from build123d import *

# Parameters (mm, degrees)
SKETCH1_R               = 6.35
BOSS_EXTRUDE1_DEPTH     = 25.4
SHELL1_T                = -0.889
FILLET1_R               = 1.27
SKETCH2_R               = 4.7625
BOSS_EXTRUDE2_DEPTH     = 10.16
CUT_EXTRUDE1_START      = -10.16
CUT_EXTRUDE1_DEPTH      = 10.16
CUT_EXTRUDE2_DEPTH      = 28.452277251
CUT_EXTRUDE2_DEPTH_BACK = 28.452277251
SKETCH4_R               = 3.048
CHAMFER2_SIZE           = 0.381
FILLET2_R               = 1.27


with BuildPart() as part:
    # Sketch1 → Boss-Extrude1 (new body)
    with BuildSketch(Plane.XY):
        Circle(SKETCH1_R)
    extrude(amount=BOSS_EXTRUDE1_DEPTH)

    # Shell1
    shell1_openings = [part.faces().sort_by_distance(p)[0] for p in [
        (0, 0, 25.4),
    ]]
    offset(amount=SHELL1_T, openings=shell1_openings, kind=Kind.INTERSECTION)

    # Fillet1
    fillet1_edges = [part.edges().sort_by_distance(p)[0] for p in [
        (-6.35, 0, 0),
    ]]
    fillet(fillet1_edges, radius=FILLET1_R)

    # Sketch2 → Boss-Extrude2 (add)
    with BuildSketch(Plane(origin=(0, 0, 0), x_dir=(-1, 0, 0), z_dir=(0, 0, -1))):
        with Locations(Location((0, 0, 0), (0, 0, 180))):
            Circle(SKETCH2_R)
    extrude(amount=BOSS_EXTRUDE2_DEPTH)

    # Sketch3 → Cut-Extrude1 (cut)
    with BuildSketch(Plane(origin=(0, 0, -10.16), x_dir=(-1, 0, 0), z_dir=(0, 0, -1)).offset(CUT_EXTRUDE1_START)):
        with BuildLine():
            Line((-1.905, 4.364903349), (-1.905, -4.364903349))
            ThreePointArc((-1.905, -4.364903349), (-4.7625, 0), (-1.905, 4.364903349))
        make_face()
        with BuildLine():
            Line((1.905, 4.364903349), (1.905, -4.364903349))
            ThreePointArc((1.905, -4.364903349), (4.7625, 0), (1.905, 4.364903349))
        make_face()
    extrude(amount=CUT_EXTRUDE1_DEPTH, mode=Mode.SUBTRACT)

    # Sketch4 → Cut-Extrude2 (cut, two sides: drawn at the far end of the back side and taken through both)
    with BuildSketch(Plane(origin=(1.905, 0, 0), x_dir=(0, 0, -1), z_dir=(1, 0, 0)).offset(-CUT_EXTRUDE2_DEPTH_BACK)):
        with Locations(Location((5.3975, 0, 0), (0, 0, 90))):
            Circle(SKETCH4_R)
    extrude(amount=CUT_EXTRUDE2_DEPTH + CUT_EXTRUDE2_DEPTH_BACK, mode=Mode.SUBTRACT)

    # Chamfer2
    chamfer2_edges = [part.edges().sort_by_distance(p)[0] for p in [
        (1.905, -3.048, -5.3975),
        (-1.905, -3.048, -5.3975),
    ]]
    chamfer(chamfer2_edges, length=CHAMFER2_SIZE)

    # Fillet2
    fillet2_edges = [part.edges().sort_by_distance(p)[0] for p in [
        (0, 4.7625, -10.16),
        (0, -4.7625, -10.16),
    ]]
    fillet(fillet2_edges, radius=FILLET2_R)


solid = part.part
Work out the finished part from the listing and answer in its coordinate system (mm). A direction names the side the tool comes from. Round coordinates to 2 decimals unless told otherwise and drop trailing zeros. Order: outer loops, then holes, each group sorted by start corner. A loop starts at its lowest first (then second) coordinate and runs counter-clockwise, first axis right, second up. Notation, with made-up numbers: M -32.5,62 L -27.5,62 A16 ccw -27.5,85 Z; hole C 6.5,59.5 d1. An arc over 180 degrees is marked long. Put each result on its own line as item: value. Start each with the question number.
Q1. Section B-B, the plane x = 0 is taken. Write down the section's boundary in (y, z), and give its area (3 significant figures).
Q2. Section C-C, the plane z = 4.5 is taken. Write down the section's boundary in (x, y), and give its area (3 significant figures).
Q3. For a pull along Y with two mould halves and no side action, classify faces 1 (the cylindrical face through (5.21, 1.64, 12.97)), 2 (the cylindrical face through (0.027, -4.762, -4.383)), 3 (the flat face through (2.2, 0.1, 0)) as pulls with the +Y half, pulls with the -Y half, needs draft (parallel to the pull), parting line crosses it, or undercut.
Q4. A tool of negligible diameter and unlimited length cuts with its end or side. For faces 4 (the flat face through (0, 0, 0.889)), 5 (the cylindrical face through (-0.027, 4.762, -4.383)), 6 (the flat face through (1.905, 0.1, -1.6)), 7 (the flat face through (-1.905, 0.1, -1.6)), from which of +Z, -Z, +X, -X, +Y, -Y can it reach the whole face along a straight path? Write none if from no direction.
Q5. Flat-ended cylindrical pins translate along their axes: pin 1 (1.5 mm diameter, centred on y = -2, z = 6.5, fed in from -X); pin 2 (2 mm diameter, centred on x = 3, z = -6.5, fed in from -Y) (3 decimals); pin 3 (1.5 mm diameter, centred on y = -0.5, z = -2.5, fed in from -X) (3 decimals). Find the tip coordinate at first contact, or state that the pin passes through.
Q6. Straight lines are drawn through the part: L1, parallel to Y at x = 0, z = 6.75; L2, parallel to Z at x = 0.35, y = 0; L3, parallel to X at y = 2.25, z = -1 (3 decimals). For each, find the intervals that lie inside material, in ascending order. Write a range as [from, to].
Findings below:
1. outline: M -6.35,1.27 A1.27 ccw -5.08,0 L -4.76,0 L -4.76,-8.89 A1.27 ccw -3.49,-10.16 L 3.49,-10.16 A1.27 ccw 4.76,-8.89 L 4.76,0 L 5.08,0 A1.27 ccw 6.35,1.27 L 6.35,25.4 L 5.46,25.4 L 5.46,0.89 L -5.46,0.89 L -5.46,25.4 L -6.35,25.4 Z; hole C 0,-5.4 d6.1
1. area: 121 mm^2
2. outline: C 0,0 d12.7; hole C 0,0 d10.92
2. area: 33.0 mm^2
3. face 1: undercut
3. face 2: pulls with the -Y half
3. face 3: needs draft
4. face 4: +Z
4. face 5: -Z, +Y
4. face 6: -Z, +X, +Y, -Y
4. face 7: -Z, -X, +Y, -Y
5. pin 1: stops at x = -6.23
5. pin 2: passes through
5. pin 3: stops at x = -1.905
6. L1: y = [-6.35, -5.46], [5.46, 6.35]
6. L2: z = [-10.16, -8.45], [-2.35, 0.89]
6. L3: x = [-1.905, 1.905]
